Check sheet for the drawn part. Datum: minimum x, y, z corner. Units: mm. Coordinates: 2 decimals unless noted, no trailing zeros. Order: outer loops, then holes, each group sorted by start corner. A loop starts at its lowest first (then second) coordinate and runs counter-clockwise, first axis right, second up. Notation, with made-up numbers: (71, -17.75) -> (125, -17.75) arc R16 ccw to (125, -11.75) -> close; hole circle Ø11 at (27, -3). An arc over 180 degrees is marked (long way). Answer as CSV lines item,"result".
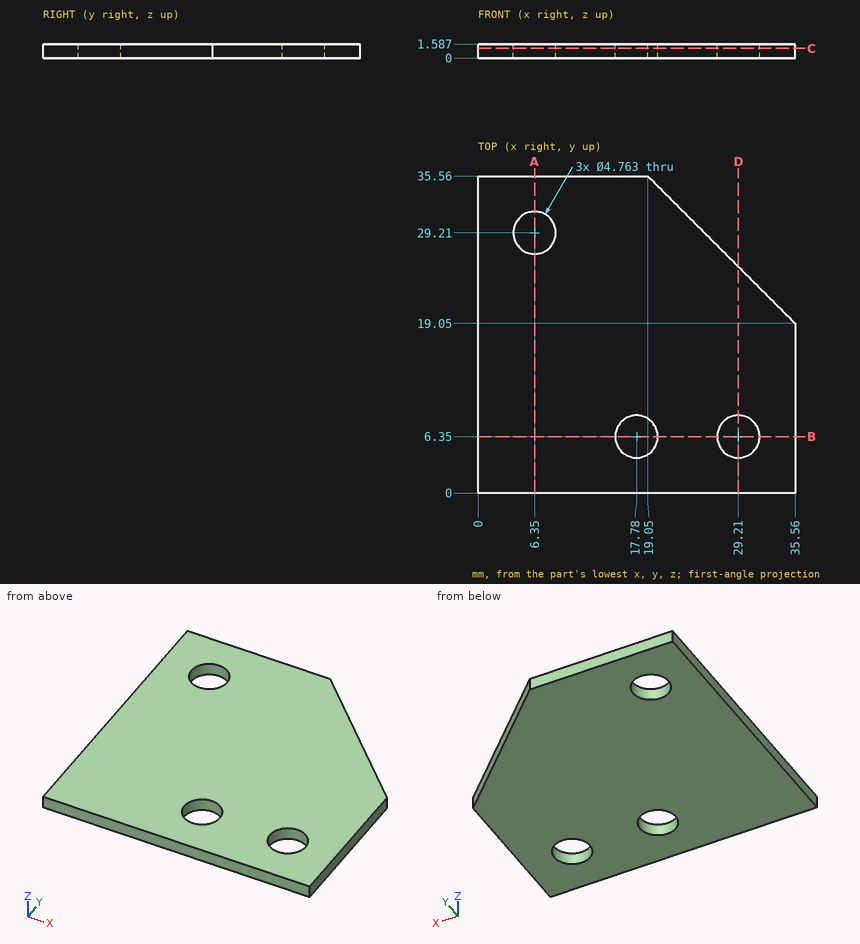
Item 1: Thickness scan on line 1 (Y direction, x = 17.78, z = 0.6); line 2 (Y direction, x = 6.35, z = 0.65); line 3 (X direction, y = 29.5, z = 0.6) (1 decimal). Record the ranges inside material, lowest first.
Answer list:
line 1,"0 to 3.97, 8.73 to 35.56"
line 2,"0 to 26.83, 31.59 to 35.56"
line 3,"0 to 4, 8.7 to 25.1"
Item 2: Depth check by flat-ended pin: pin 1 Ø4.5 at (x, y) = (6.35, 29.21) entering from -Z. Enter the tip coordinate at first touch or a pass-through.
Answer list:
pin 1,"through"
Item 3: Section check B-B, the plane y = 6.35. Record the boundary of the cut face in (x, z).
Answer list:
outline,"(0, 0) -> (15.4, 0) -> (15.4, 1.59) -> (0, 1.59) -> close; (20.16, 0) -> (26.83, 0) -> (26.83, 1.59) -> (20.16, 1.59) -> close; (31.59, 0) -> (35.56, 0) -> (35.56, 1.59) -> (31.59, 1.59) -> close"
Item 4: Section check A-A, the plane x = 6.35. Record the boundary of the cut face in (y, z).
Answer list:
outline,"(0, 0) -> (26.83, 0) -> (26.83, 1.59) -> (0, 1.59) -> close; (31.59, 0) -> (35.56, 0) -> (35.56, 1.59) -> (31.59, 1.59) -> close"
Item 5: Section check C-C, the plane z = 1.1. Record the boundary of the cut face in (x, y).
Answer list:
outline,"(0, 0) -> (35.56, 0) -> (35.56, 19.05) -> (19.05, 35.56) -> (0, 35.56) -> close; hole circle Ø4.76 at (6.35, 29.21); hole circle Ø4.76 at (17.78, 6.35); hole circle Ø4.76 at (29.21, 6.35)"
Item 6: Section check D-D, the plane x = 29.21. Record the boundary of the cut face in (y, z).
Answer list:
outline,"(0, 0) -> (3.97, 0) -> (3.97, 1.59) -> (0, 1.59) -> close; (8.73, 0) -> (25.4, 0) -> (25.4, 1.59) -> (8.73, 1.59) -> close"
